Could you check a few things on this drawing? It's one solid part, dimensions in mm from its lowest x, y, z. Round coordinates to 2 decimals unless told otherwise and drop trailing zeros. Order: outer loops, then holes, each group sorted by start corner. A loop starts at its lowest first (then second) coordinate and runs counter-clockwise, first axis right, second up.
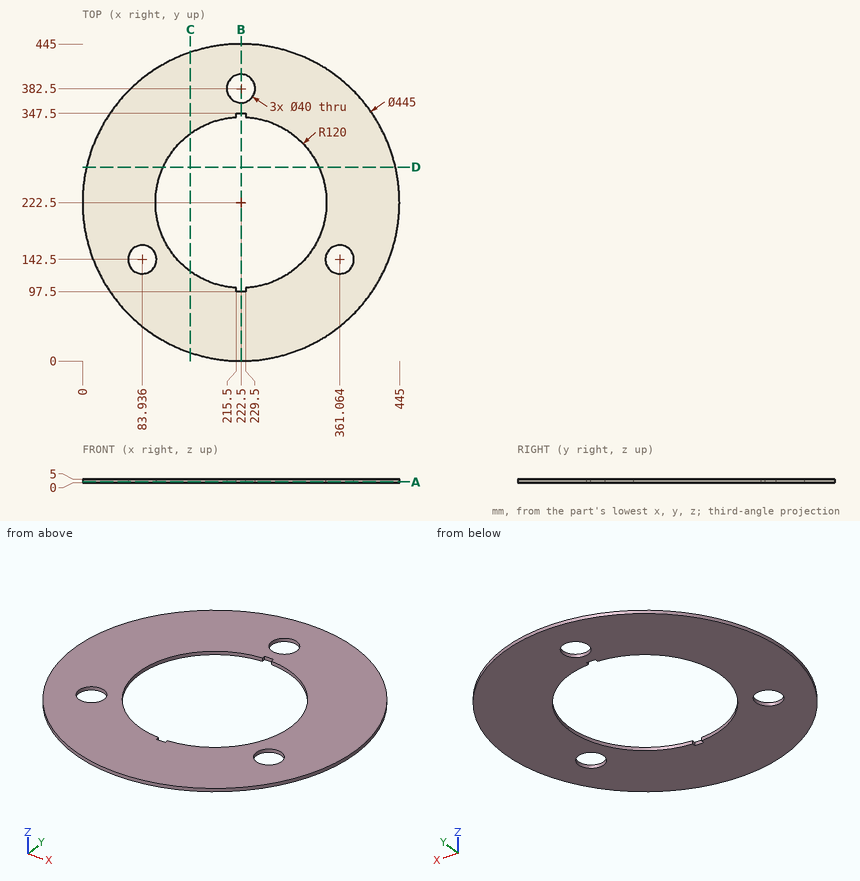
1) If we section it at B-B (x = 222.5): Write out the boundary of the cut face in (y, z).
2) I need wall thicknesses on line 1 (X direction, y = 224.5, z = 1.1); line 2 (X direction, y = 158, z = 1.85) (1 decimal); line 3 (Y direction, x = 377, z = 2.75) (1 decimal). Which ranges of each line are inside material? Lowest first, please.
3) If we section it at A-A (z = 1.1): Write out the boundary of the cut face in (x, y).
4) If we section it at C-C (x = 151.5): Write out the boundary of the cut face in (y, z).
5) I'm going to push flat-ended pins straight in: pin 1 (1 mm diameter, centred on x = 286.5, z = 1.5, fed in from +Y); pin 2 (1.5 mm diameter, centred on y = 346, z = 3.5, fed in from +X); pin 3 (2.5 mm diameter, centred on y = 100.5, z = 3.5, fed in from +X). Where does each tip first touch, or does it pass through?
6) If we section it at D-D (y = 272): Write out the boundary of the cut face in (x, z) (3 decimals), plus the area to 3 significant figures.
Solutions:
1. outline: (0, 0) - (97.5, 0) - (97.5, 5) - (0, 5) - close; (347.5, 0) - (362.5, 0) - (362.5, 5) - (347.5, 5) - close; (402.5, 0) - (445, 0) - (445, 5) - (402.5, 5) - close
2. line 1: x = 0.01 to 102.52, 342.48 to 444.99
2. line 2: x = 9.6 to 71.3, 96.6 to 121.3, 323.7 to 348.4, 373.7 to 435.4
2. line 3: y = 62.4 to 130.4, 154.6 to 382.6
3. outline: circle Ø445 at (222.5, 222.5); hole circle Ø40 at (83.94, 142.5); hole circle Ø40 at (222.5, 382.5); hole (215.5, 97.5) - (229.5, 97.5) - (229.5, 102.7) arc R120 ccw to (342.5, 222.5) arc R120 ccw to (229.5, 342.3) - (229.5, 347.5) - (215.5, 347.5) - (215.5, 342.3) arc R120 ccw to (215.5, 102.7) - close; hole circle Ø40 at (361.06, 142.5)
4. outline: (11.63, 0) - (125.76, 0) - (125.76, 5) - (11.63, 5) - close; (319.24, 0) - (433.37, 0) - (433.37, 5) - (319.24, 5) - close
5. pin 1: stops at y = 435.75
5. pin 2: stops at x = 408.08
5. pin 3: stops at x = 409.38
6. outline: (5.576, 0) - (113.185, 0) - (113.185, 5) - (5.576, 5) - close; (331.815, 0) - (439.424, 0) - (439.424, 5) - (331.815, 5) - close
6. area: 1,080 mm2
